The figure shows three views and two pictorial views of one solid part (mm, origin at its lowest corner). Answer the questions. A direction names the side the tool comes from. Coordinates: 2 decimals unless noted, no trailing zeros. Write each loop counter-clockwise with the first axis right and the second up, starting at its lowest first coordinate (ties: lowest second). Pieces come first, ordered by that corner, then holes. Notation, with made-up numbers: M 49.5,34 L 64.5,34 A27 cw 64.5,54 Z; hole C 53,72.5 d4. An arc over 180 degrees is marked long. Write item = value, one per line. Start each with the question number.
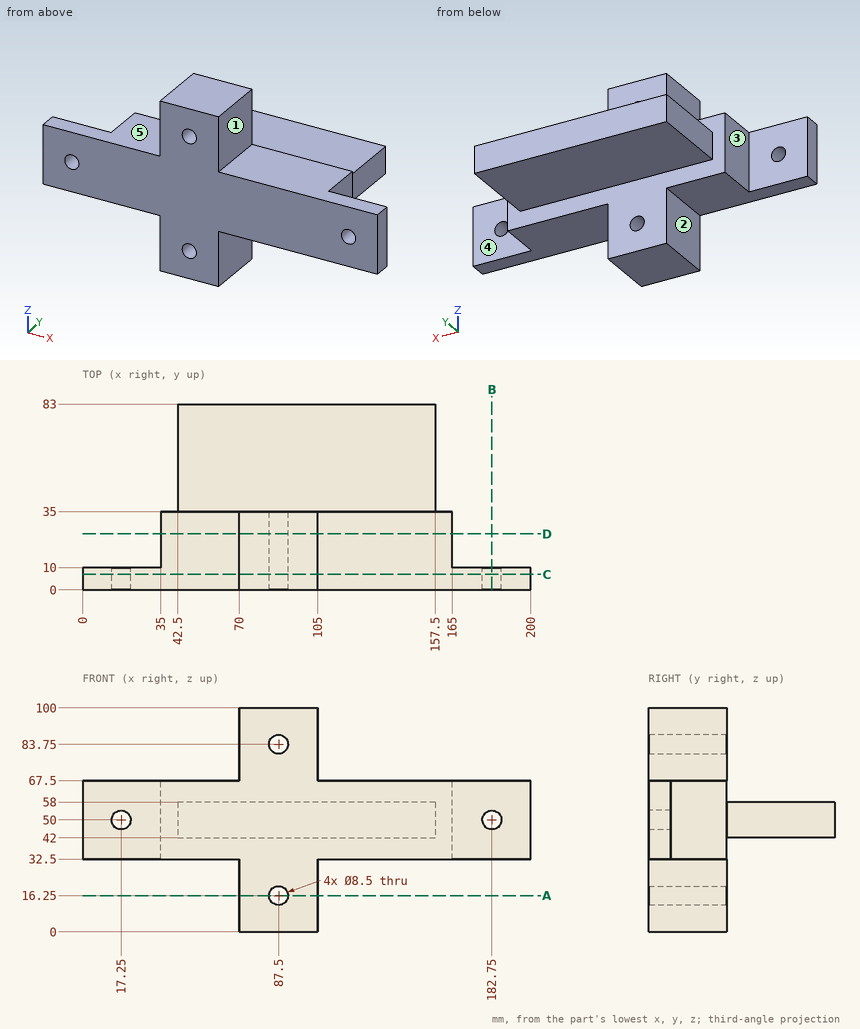
1. Straight lines are drawn through the part: L1, parallel to Z at x = 87.5, y = 25.5; L2, parallel to X at y = 3.25, z = 50; L3, parallel to X at y = 21.5, z = 16.25. For each, find the intervals that lie inside material, in ascending order. Write a range as [from, to].
2. The part is cut by section B-B, the plane x = 182.75. Write down the section's boundary in (y, z).
3. For the marked faces 1, 2, 3, 4 and 5, determine the directions among +Z, -Z, +X, -X, +Y, -Y from which every point of the face is accessible in a straight line to the end or side of a thin tool.
4. The part is cut by section D-D, the plane y = 25. Write down the section's boundary in (x, z).
5. Each of these flat-tipped pins is pushed along its axis until it touches: pin 1 (5 mm diameter, centred on y = 14, z = 89, fed in from +X); pin 2 (12.5 mm diameter, centred on y = 18.5, z = 41.5, fed in from +X); pin 3 (10 mm diameter, centred on y = 22, z = 77, fed in from -X); pin 4 (8 mm diameter, centred on y = 49, z = 63.5, fed in from -X). Where does it stop, or does it pass through?
6. The part is cut by section A-A, the plane z = 16.25. Write down the section's boundary in (x, y).
7. The part is cut by section C-C, the plane y = 7. Write down the section's boundary in (x, z), and give its area (3 significant figures).
Solution:
q1.L1 = [0, 12], [20.5, 79.5], [88, 100]
q1.L2 = [0, 13], [21.5, 178.5], [187, 200]
q1.L3 = [70, 83.25], [91.75, 105]
q2.outline = M 0,32.5 L 10,32.5 L 10,45.75 L 0,45.75 Z; M 0,54.25 L 10,54.25 L 10,67.5 L 0,67.5 Z
q3.face_1 = +Z, +X, +Y, -Y
q3.face_2 = -Z, -X, +Y, -Y
q3.face_3 = +Z, -Z, -X, +Y
q3.face_4 = +Z, -Z, +X, +Y
q3.face_5 = +Z, -X, +Y, -Y
q4.outline = M 35,32.5 L 70,32.5 L 70,0 L 105,0 L 105,32.5 L 165,32.5 L 165,67.5 L 105,67.5 L 105,100 L 70,100 L 70,67.5 L 35,67.5 Z; hole C 87.5,16.25 d8.5; hole C 87.5,83.75 d8.5
q5.pin_1 = 105
q5.pin_2 = 165
q5.pin_3 = 70
q5.pin_4 = through
q6.outline = M 70,0 L 83.25,0 L 83.25,35 L 70,35 Z; M 91.75,0 L 105,0 L 105,35 L 91.75,35 Z
q7.outline = M 0,32.5 L 70,32.5 L 70,0 L 105,0 L 105,32.5 L 200,32.5 L 200,67.5 L 105,67.5 L 105,100 L 70,100 L 70,67.5 L 0,67.5 Z; hole C 17.25,50 d8.5; hole C 87.5,16.25 d8.5; hole C 87.5,83.75 d8.5; hole C 182.75,50 d8.5
q7.area = 9,050 mm^2
